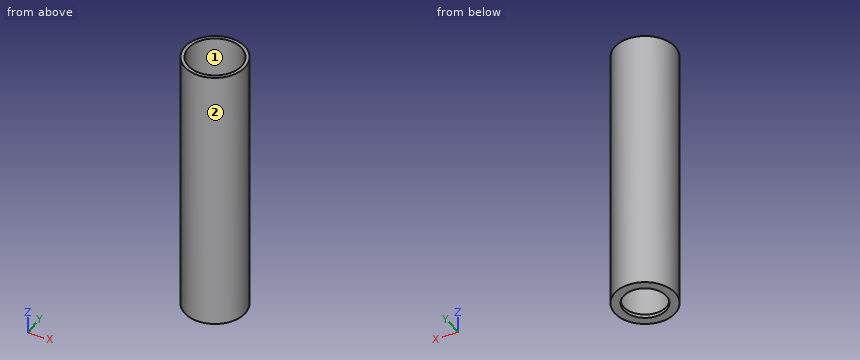
```python
from build123d import *

# Parameters (mm, degrees)
ESQUISSE1_R             = 17
BOSS_EXTRU_1_DEPTH      = 2
ESQUISSE2_R             = 17
ESQUISSE2_R_2           = 15
BOSS_EXTRU_2_DEPTH      = 150
ESQUISSE3_R             = 12
ENL_V_MAT_EXTRU_1_DEPTH = 150


with BuildPart() as part:
    # Esquisse1 → Boss.-Extru.1 (new body)
    with BuildSketch(Plane.XY):
        Circle(ESQUISSE1_R)
    extrude(amount=BOSS_EXTRU_1_DEPTH)

    # Esquisse2 → Boss.-Extru.2 (add)
    with BuildSketch(Plane.XY.offset(2)):
        Circle(ESQUISSE2_R)
        Circle(ESQUISSE2_R_2, mode=Mode.SUBTRACT)
    extrude(amount=BOSS_EXTRU_2_DEPTH)

    # Esquisse3 → Enlèv. mat.-Extru.1 (cut)
    with BuildSketch(Plane(origin=(0, 0, 0), x_dir=(-1, 0, 0), z_dir=(0, 0, -1))):
        Circle(ESQUISSE3_R)
    extrude(amount=-ENL_V_MAT_EXTRU_1_DEPTH, mode=Mode.SUBTRACT)


solid = part.part
```
Check sheet for the modelled part. Datum: model origin and axes. Units: mm. Face numbers are marked on the shaded views. A direction names the side the tool comes from. Coordinates: 2 decimals unless noted, no trailing zeros. Write each loop counter-clockwise with the first axis right and the second up, starting at its lowest first coordinate (ties: lowest second). Pieces come first, ordered by that corner, then holes. Notation, with made-up numbers: M 81.25,28.25 L 118.25,28.25 A4 cw 118.25,33.25 Z; hole C 31.5,-35 d6. An arc over 180 degrees is marked long. Write item = value, one per line. Start each with the question number.
1. Sectioned sample at C-C (z = 9.5). Record the cut outline in (x, y), then the cut area to 3 significant figures.
2. Thickness scan on probe 1 along Y at (x, z) = (0, 1.1); probe 2 along Y at (x, z) = (0, 72); probe 3 along Z at (x, y) = (2.5, -13). Record the ranges inside material, lowest first.
3. Tool access check on the marked faces 1 and 2. Record the directions out of +Z, -Z, +X, -X, +Y, -Y that give a thin tool (end or side, any length) a straight path to the whole face; none if there is none.
4. Sectioned sample at A-A (x = 0). Record the cut outline in (y, z), then the cut area to 3 significant figures.
5. Go/stop test with flat-tipped pins: pin 1 (1.5 mm diameter, centred on x = 7, z = 30, fed in from -Y); pin 2 (1 mm diameter, centred on y = -8.5, z = 124.5, fed in from +X); pin 3 (3 mm diameter, centred on x = 5.5, z = 40, fed in from -Y). Record where each tip stops, or that it passes through.
The answers:
q1.outline = C 0,0 d34; hole C 0,0 d30
q1.area = 201 mm²
q2.probe_1 = -17 to -12, 12 to 17
q2.probe_2 = -17 to -15, 15 to 17
q2.probe_3 = 0 to 2
q3.face_1 = +Z
q3.face_2 = +Z, -Z
q4.outline = M -17,0 L -12,0 L -12,2 L -15,2 L -15,152 L -17,152 Z; M 12,0 L 17,0 L 17,152 L 15,152 L 15,2 L 12,2 Z
q4.area = 620 mm²
q5.pin_1 = -15.81
q5.pin_2 = 15
q5.pin_3 = -16.52
